Source: CAD feature listing. Evaluate the final solid. Frame: model axes, mm. Face numbers are marked on the shaded views. Coordinates: 2 decimals unless noted, no trailing zeros. Loops run counter-clockwise (first coordinate to the right, second up) from the corner with the lowest first, then second, coordinate; pieces in that order, holes last.
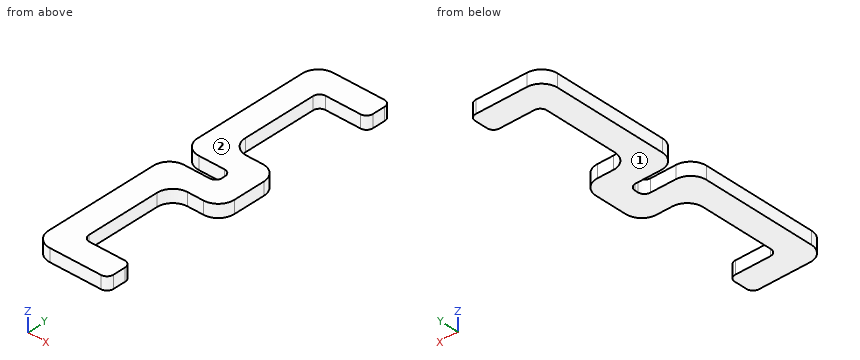
from build123d import *

# Parameters (mm, degrees)
F1_DEPTH = 4


with BuildPart() as f1:
    # F0 (on Top) → F1 (new body)
    with BuildSketch(Plane.XY):
        with BuildLine():
            ThreePointArc((10.238371, 46), (9.652584, 47.414214), (8.238371, 48))
            Line((8.238371, 48), (-7.761629, 48))
            ThreePointArc((-7.761629, 48), (-11.297163, 46.535534), (-12.761629, 43))
            Line((-12.761629, 43), (-12.761629, 7.5))
            ThreePointArc((-12.761629, 7.5), (-11.297163, 3.964466), (-7.761629, 2.5))
            Line((-7.761629, 2.5), (0.238371, 2.5))
            ThreePointArc((0.238371, 2.5), (1.652584, 1.914214), (2.238371, 0.5))
            Line((2.238371, 0.5), (2.238371, -0.5))
            ThreePointArc((2.238371, -0.5), (1.652584, -1.914214), (0.238371, -2.5))
            Line((0.238371, -2.5), (-7.761629, -2.5))
            ThreePointArc((-7.761629, -2.5), (-11.297163, -3.964466), (-12.761629, -7.5))
            Line((-12.761629, -7.5), (-12.761629, -43))
            ThreePointArc((-12.761629, -43), (-11.297163, -46.535534), (-7.761629, -48))
            Line((-7.761629, -48), (8.238371, -48))
            ThreePointArc((8.238371, -48), (9.652584, -47.414214), (10.238371, -46))
            Line((10.238371, -46), (10.238371, -42))
            ThreePointArc((10.238371, -42), (9.652584, -40.585786), (8.238371, -40))
            Line((8.238371, -40), (-2.761629, -40))
            ThreePointArc((-2.761629, -40), (-4.175843, -39.414214), (-4.761629, -38))
            Line((-4.761629, -38), (-4.761629, -15))
            ThreePointArc((-4.761629, -15), (-3.297163, -11.464466), (0.238371, -10))
            Line((0.238371, -10), (5.238371, -10))
            ThreePointArc((5.238371, -10), (8.773904, -8.535534), (10.238371, -5))
            Line((10.238371, -5), (10.238371, 5))
            ThreePointArc((10.238371, 5), (8.773904, 8.535534), (5.238371, 10))
            Line((5.238371, 10), (0.238371, 10))
            ThreePointArc((0.238371, 10), (-3.297163, 11.464466), (-4.761629, 15))
            Line((-4.761629, 15), (-4.761629, 38))
            ThreePointArc((-4.761629, 38), (-4.175843, 39.414214), (-2.761629, 40))
            Line((-2.761629, 40), (8.238371, 40))
            ThreePointArc((8.238371, 40), (9.652584, 40.585786), (10.238371, 42))
            Line((10.238371, 42), (10.238371, 46))
        make_face()
    extrude(amount=F1_DEPTH)


solid = f1.part
Q1. Section A-A, the plane x = -6.5. Return the cut outline in (y, z).
Q2. Section D-D, the plane x = -1.75. Return the cut outline in (y, z), plus the area to 3 significant figures.
Q3. Section B-B, the plane x = 3.75. Return the cut outline in (y, z), plus the area to 3 significant figures.
Q4. Line query: line 1 along Y through (x, z) = (5.25, 1.5); line 2 along Y through (x, z) = (-7.75, 2.35); line 3 along Y through (x, z) = (-1.25, 2.1). Output: solid intervals per line, ascending.
Q5. Contact query for flat-ended pins moving along their axis: pin 1 Ø3 at (x, y) = (-2, -37.5) entering from -Z; pin 2 Ø1.5 at (y, z) = (-29.5, 3) entering from +X; pin 3 Ø0.5 at (y, z) = (0, 2) entering from -X. Output: stop coordinate, or through.
Q6. Draft query along Z for the marked faces 1 and 2. Return one class per face: +Z half, -Z half, draft (parallel to the pull), parting line (faces both ways), or undercut.
Derived:
1. outline: (-48, 0) - (-2.5, 0) - (-2.5, 4) - (-48, 4) - close; (2.5, 0) - (48, 0) - (48, 4) - (2.5, 4) - close
2. outline: (-48, 0) - (-40, 0) - (-40, 4) - (-48, 4) - close; (-10.41, 0) - (-2.5, 0) - (-2.5, 4) - (-10.41, 4) - close; (2.5, 0) - (10.41, 0) - (10.41, 4) - (2.5, 4) - close; (40, 0) - (48, 0) - (48, 4) - (40, 4) - close
2. area: 127 mm2
3. outline: (-48, 0) - (-40, 0) - (-40, 4) - (-48, 4) - close; (-10, 0) - (10, 0) - (10, 4) - (-10, 4) - close; (40, 0) - (48, 0) - (48, 4) - (40, 4) - close
3. area: 144 mm2
4. line 1: y = -48 to -40, -10 to 10, 40 to 48
4. line 2: y = -48 to -2.5, 2.5 to 48
4. line 3: y = -48 to -40, -10.23 to -2.5, 2.5 to 10.23, 40 to 48
5. pin 1: passes through
5. pin 2: stops at x = -4.76
5. pin 3: stops at x = 2.24
6. face 1: -Z half
6. face 2: +Z half
